Verification items for the finished model (mm, model axes). Face numbers are marked on the shaded views. A direction names the side the tool comes from. Round coordinates to 2 decimals unless told otherwise and drop trailing zeros. Write each loop counter-clockwise with the first axis right and the second up, starting at its lowest first coordinate (ties: lowest second). Pieces come first, ordered by that corner, then holes. Notation, with made-up numbers: M 83,-11.75 L 89,-11.75 A24 cw 89,-0.75 Z; hole C 26.5,78.25 d2. An arc over 180 degrees is marked long. One line per item, written item: value. Start each with the question number.
Item 1: Thickness scan on probe 1 along Y at (x, z) = (2.5, 1.5); probe 2 along Y at (x, z) = (-8, 2.75); probe 3 along Z at (x, y) = (-29.5, -22.5). Record the ranges inside material, lowest first. Write a range as from..to.
Item 2: Gauge pin test, flat ends, axial feed: pin 1 (1.6 mm diameter, centred on x = -3.5, z = 1, fed in from +Y); pin 2 (2.5 mm diameter, centred on x = -31.5, y = -24.5, fed in from +Z); pin 3 (5 mm diameter, centred on y = -25, z = 8.5, fed in from +X); pin 4 (1.2 mm diameter, centred on x = 22.4, y = 9.76, fed in from -Z). Record the tip position at first contact, or that the pin passes through.
Item 3: Section check B-B, the plane x = -32. Record the cut outline in (y, z), then the cut area to 3 significant figures.
Item 4: Section check A-A, the plane z = 6.25. Record the cut outline in (x, y), then the cut area to 3 significant figures.
Item 5: Tool access check on the marked faces 1, 2, 3, 4 and 5. Record the directions out of +Z, -Z, +X, -X, +Y, -Y that give a thin tool (end or side, any length) a straight path to the whole face; none if there is none.
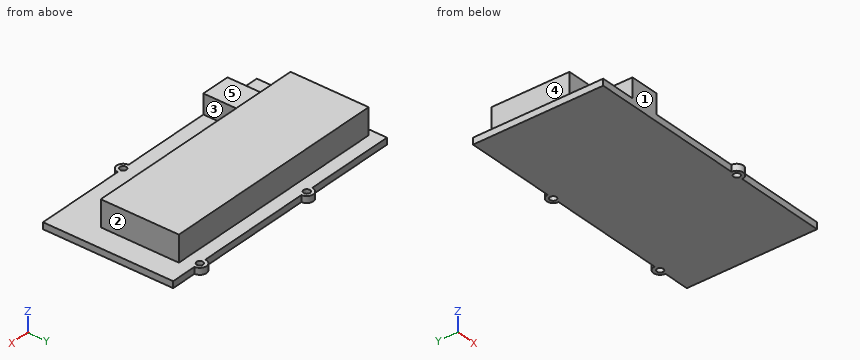
from build123d import *

# Parameters (mm, degrees)
ESQUISSE1_R        = 1
BOSS_EXTRU_1_DEPTH = 2
ESQUISSE2_W        = 71
ESQUISSE2_H        = 24
BOSS_EXTRU_3_DEPTH = 8
ESQUISSE4_W        = 9
ESQUISSE4_H        = 12
BOSS_EXTRU_4_DEPTH = 6


with BuildPart() as part:
    # Esquisse1 → Boss.-Extru.1 (new body)
    with BuildSketch(Plane.XY):
        with BuildLine():
            Line((-47.60021768, -30.24324737), (0.39978232, -30.24324737))
            ThreePointArc((0.39978232, -30.24324737), (2.39978232, -32.24324737), (4.39978232, -30.24324737))
            Line((4.39978232, -30.24324737), (32.39978232, -30.24324737))
            Line((32.39978232, -30.24324737), (32.39978232, 9.75675263))
            Line((32.39978232, 9.75675263), (24.39978232, 9.75675263))
            ThreePointArc((24.39978232, 9.75675263), (22.39978232, 11.75675263), (20.39978232, 9.75675263))
            Line((20.39978232, 9.75675263), (-15.60021768, 9.75675263))
            ThreePointArc((-15.60021768, 9.75675263), (-17.60021768, 11.75675263), (-19.60021768, 9.75675263))
            Line((-19.60021768, 9.75675263), (-47.60021768, 9.75675263))
            Line((-47.60021768, 9.75675263), (-47.60021768, -30.24324737))
        make_face()
        with Locations((22.39978232, 9.75675263)):
            Circle(ESQUISSE1_R, mode=Mode.SUBTRACT)
        with Locations((-17.60021768, 9.75675263)):
            Circle(ESQUISSE1_R, mode=Mode.SUBTRACT)
        with Locations((2.39978232, -30.24324737)):
            Circle(ESQUISSE1_R, mode=Mode.SUBTRACT)
    extrude(amount=BOSS_EXTRU_1_DEPTH)

    # Esquisse2 → Boss.-Extru.3 (add)
    with BuildSketch(Plane.XY.offset(2)):
        with Locations((-10.10021768, -6.24324737)):
            Rectangle(ESQUISSE2_W, ESQUISSE2_H)
    extrude(amount=BOSS_EXTRU_3_DEPTH)

    # Esquisse4 → Boss.-Extru.4 (add)
    with BuildSketch(Plane.XY.offset(2)):
        with Locations((-32.10021768, -24.24324737)):
            Rectangle(ESQUISSE4_W, ESQUISSE4_H)
    extrude(amount=BOSS_EXTRU_4_DEPTH)


solid = part.part
Response values:
1. probe 1: y = -32.24..-31.24, -29.25..9.76
1. probe 2: y = -18.24..5.76
1. probe 3: z = 0..8
2. pin 1: stops at y = 9.76
2. pin 2: stops at z = 8
2. pin 3: stops at x = -27.6
2. pin 4: passes through
3. outline: M -30.24,0 L 9.76,0 L 9.76,2 L 5.76,2 L 5.76,10 L -18.24,10 L -18.24,8 L -30.24,8 Z
3. area: 344 mm2
4. outline: M -45.6,-18.24 L -36.6,-18.24 L -36.6,-30.24 L -27.6,-30.24 L -27.6,-18.24 L 25.4,-18.24 L 25.4,5.76 L -45.6,5.76 Z
4. area: 1,810 mm2
5. face 1: +Z, -Z, -X, -Y
5. face 2: +Z, +X, +Y, -Y
5. face 3: +Z, +X, -Y
5. face 4: +Z, -X, +Y, -Y
5. face 5: +Z, +X, -X, -Y
